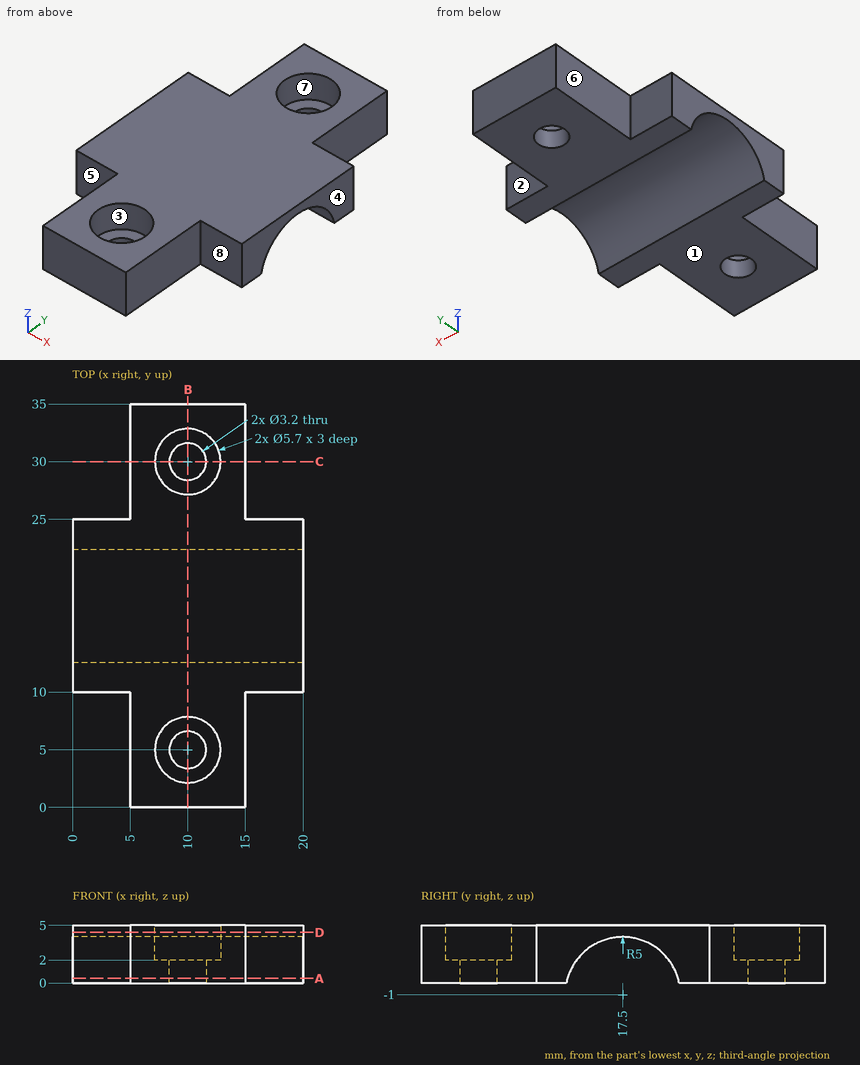
Could you check a few things on this drawing? It's one solid part, dimensions in mm from its lowest x, y, z. A direction names the side the tool comes from. Coordinates: 2 decimals unless noted, no trailing zeros. Write each loop counter-clockwise with the first axis right and the second up, starting at its lowest first coordinate (ties: lowest second). Pieces come first, ordered by that corner, then holes. Notation, with made-up numbers: (-8.5, -13) - (47.5, -13) arc R30 ccw to (47.5, 10) - close; hole circle Ø9 at (-22, 49.5). An arc over 180 degrees is marked (long way). Put each result on its own line as item: value. Start each with the question number.
Q1. Please list where these lines run through material, in increasing order: L1, parallel to Y at x = 10, z = 4.45; L2, parallel to Y at x = 9.25, z = 4.85; L3, parallel to Y at x = 10, z = 0.8.
Q2. Which directions (+Z, -Z, +X, -X, +Y, -Y) give clear straight access to the entire face, cutting with the end or side of a thin tool? Please do the marked faces 4, 5, 6, 7 and 8.
Q3. Thinking about a two-plate mould opening in Y: for the marked faces 1, 2 and 3, which applies, pulls with the +Y half, pulls with the -Y half, needs draft (parallel to the pull), parting line crosses it, or undercut?
Q4. I want a section at B-B on x = 10. Write out the boundary of the cut face in (y, z).
Q5. I'm going to push flat-ended pins straight in: P1, Ø1.7, axis at x = 9, y = 6, coming from the +Z side; P2, Ø2.5, axis at x = 10, y = 30, coming from the -Z side; P3, Ø6, axis at x = 11.5, y = 19, coming from the -Z side; P4, Ø2.5, axis at y = 31.5, z = 2.5, coming from the -X side. Where does each tip first touch, or does it pass through?
Q6. I want a section at A-A on z = 0.4. Write out the boundary of the cut face in (x, y), plus the area to 3 significant figures.
Q7. I want a section at D-D on z = 4.4. Write out the boundary of the cut face in (x, y), plus the area to 3 significant figures.
Q8. I want a section at C-C on y = 30. Write out the boundary of the cut face in (x, z).
Checks:
1. L1: 0 to 2.15, 7.85 to 27.15, 32.85 to 35
1. L2: 0 to 2.25, 7.75 to 27.25, 32.75 to 35
1. L3: 0 to 3.4, 6.6 to 12.84, 22.16 to 28.4, 31.6 to 35
2. face 4: +Z, -Z, +X, +Y, -Y
2. face 5: +Z, -Z, -X, -Y
2. face 6: +Z, -Z, -X, +Y
2. face 7: +Z
2. face 8: +Z, -Z, +X, -Y
3. face 1: needs draft
3. face 2: pulls with the +Y half
3. face 3: undercut
4. outline: (0, 0) - (3.4, 0) - (3.4, 2) - (2.15, 2) - (2.15, 5) - (0, 5) - close; (6.6, 0) - (12.6, 0) arc R5 cw to (22.4, 0) - (28.4, 0) - (28.4, 2) - (27.15, 2) - (27.15, 5) - (7.85, 5) - (7.85, 2) - (6.6, 2) - close; (31.6, 0) - (35, 0) - (35, 5) - (32.85, 5) - (32.85, 2) - (31.6, 2) - close
5. P1: z = 2
5. P2: through
5. P3: z = 1.18
5. P4: x = 5
6. outline: (0, 10) - (5, 10) - (5, 0) - (15, 0) - (15, 10) - (20, 10) - (20, 12.7) - (0, 12.7) - close; (0, 22.3) - (20, 22.3) - (20, 25) - (15, 25) - (15, 35) - (5, 35) - (5, 25) - (0, 25) - close; hole circle Ø3.2 at (10, 5); hole circle Ø3.2 at (10, 30)
6. area: 292 mm²
7. outline: (0, 10) - (5, 10) - (5, 0) - (15, 0) - (15, 10) - (20, 10) - (20, 25) - (15, 25) - (15, 35) - (5, 35) - (5, 25) - (0, 25) - close; hole circle Ø5.7 at (10, 5); hole circle Ø5.7 at (10, 30)
7. area: 449 mm²
8. outline: (5, 0) - (8.4, 0) - (8.4, 2) - (7.15, 2) - (7.15, 5) - (5, 5) - close; (11.6, 0) - (15, 0) - (15, 5) - (12.85, 5) - (12.85, 2) - (11.6, 2) - close
